Autodesk Inventor part; units mm, degrees
ref_plane "YZ Plane" through (0, 0, 0) normal (1, 0, 0) x (0, 1, 0)
ref_plane "XZ Plane" through (0, 0, 0) normal (0, 1, 0) x (-1, 0, 0)
ref_plane "XY Plane" through (0, 0, 0) normal (0, 0, 1) x (1, 0, 0)
sketch "Sketch1" plane through (0, 0, 0) normal (0, 1, 0) x (-1, 0, 0)
  line L0 (10.07, 20.05) -> (-10.07, 20.05)
  line L1 (-10.07, 20.05) -> (-10.07, -20.05)
  line L2 (-10.07, -20.05) -> (10.07, -20.05)
  line L3 (10.07, -20.05) -> (10.07, 20.05)
  point P0 (0, 0)
  dimension "d0" = 40.1
  dimension "d1" = 20.14
  dimension "d2" = 10.07
  dimension "d3" = 20.05
extrude "Plate1" add sketch "Sketch1" along normal blind 1.5
sketch "Sketch2" plane through (10.07, 0, 21.55) normal (0, 0, -1) x (-1, 0, 0)
  line L0 (20.14, 0) -> (0, 0)
  line L1 (0, 0) -> (0, 60)
  line L2 (0, 60) -> (20.14, 60)
  line L3 (20.14, 60) -> (20.14, 0)
edge flange "Flange1" height 60 angle 90 thickness 1.5 bend radius 0.31 thickness toward (0, 0, -1) relief tear relief width 1.5 relief depth 0.75 corner gap 0.31 corner form 0 edges at (0, 1.5, 20.05) (0, 1.5, -20.05) wall of the first edge with corners at (-10.07, 0, 21.55) (10.07, 0, 21.55) (10.07, 60, 21.55) (-10.07, 60, 21.55)
bend "Bend1"
corner "Corner1"
sketch "Sketch15" plane through (10.07, 60, -21.55) normal (0, 0, -1) x (-1, 0, 0)
  circle A0 centre (2.545, -12.76) radius 0.7835
  circle A1 centre (17.595, -12.76) radius 0.7835
  circle A2 centre (2.545, -27.86) radius 0.7835
  circle A3 centre (17.595, -27.86) radius 0.7835
  point P0 (10.07, -60)
hole "Hole9" at (7.525, 47.24, -21.55) at (-7.525, 47.24, -21.55) at (7.525, 32.14, -21.55) at (-7.525, 32.14, -21.55) direction (0, 0, 1) diameter 2.1 depth 1.5
sketch "Sketch16" plane through (-10.07, 60, 21.55) normal (0, 0, 1) x (1, 0, 0)
  circle A0 centre (18.07, -7.16) radius 0.7835
  circle A1 centre (2.07, -7.16) radius 0.7835
  circle A2 centre (3.07, -20.38) radius 0.7835
  circle A3 centre (17.07, -20.38) radius 0.7835
  circle A4 centre (10.07, -27.68) radius 0.7835
  point P0 (10.07, -60)
hole "Hole10" at (-8, 52.84, 21.55) at (8, 52.84, 21.55) at (-7, 39.62, 21.55) at (7, 39.62, 21.55) at (0, 32.32, 21.55) direction (0, 0, -1) diameter 2.1 depth 1.5
sketch "Sketch17" plane through (-10.07, 60, 21.55) normal (0, 0, 1) x (1, 0, 0)
  point P0 (10.07, -60)
sketch "Sketch18" plane through (-10.07, 60, 21.55) normal (0, 0, 1) x (1, 0, 0)
  point P0 (10.07, -60)
sketch "Sketch19" plane through (-10.07, 60, 21.55) normal (0, 0, 1) x (1, 0, 0)
  circle A0 centre (10.07, -0.26) radius 6
  point P0 (10.07, -60)
sketch "Sketch20" plane through (10.07, 60, -21.55) normal (0, 0, -1) x (-1, 0, 0)
  circle A0 centre (10.07, -0.26) radius 6
  point P0 (10.07, -60)
sketch "Sketch21" plane through (0, 0, 0) normal (0, -1, 0) x (1, 0, 0)
  circle A0 centre (4.76, 2.25) radius 1.5
  circle A1 centre (4.76, -13.05) radius 1.5
  circle A2 centre (-5.38, -13.05) radius 1.5
  circle A3 centre (-5.38, 2.25) radius 1.5
  point P0 (0, 0)
fillet "Corner Round1" radius 1 4 edges at (-10.07, 60, 20.8) (-10.07, 60, -20.8) (10.07, 60, -20.8) (10.07, 60, 20.8)
hole "Hole11" at (-5.38, 0, -13.05) at (4.76, 0, -13.05) at (-5.38, 0, 2.25) at (4.76, 0, 2.25) direction (0, 1, 0) diameter 3.1 depth 1.5
hole "Hole12" at (0, 59.74, 21.55) direction (0, 0, -1) diameter 13.5 depth 1.5
hole "Hole13" at (0, 59.74, -21.55) direction (0, 0, 1) diameter 13.5 depth 1.5
equation "\"d96\" = Thickness"
equation "\"d103\" = Thickness"
equation "\"d117\" = Thickness"
equation "\"d124\" = Thickness"
equation "\"d131\" = Thickness"
equation "\"d4\" = Thickness"
equation "\"d5\" = BendReliefWidth"
equation "\"d6\" = BendReliefDepth"
equation "\"d7\" = MinimumRemnant"
equation "\"d8\" = TransitionRadius"
equation "\"d11\" = BendRadius"
equation "\"d12\" = CornerReliefSize"
equation "\"d13\" = GapSize"
equation "\"d14\" = JacobiRadiusSize"
equation "\"BendReliefWidth\" = Thickness"
equation "\"BendReliefDepth\" = 0.5 * Thickness"
equation "\"CornerReliefSize\" = 4 * Thickness"
equation "\"MinimumRemnant\" = 2 * Thickness"
equation "\"TransitionRadius\" = BendRadius"
equation "\"JacobiRadiusSize\" = BendRadius"
equation "\"GapSize\" = Thickness"
properties part number "axis_25_top_frame" material "Aluminum 6061-AHC"
Here's how the part is built. I have some questions about the finished solid (model axes, mm). A direction names the side the tool comes from. Give positions to 0.01 mm unless a question says otherwise; leave off trailing zeros. Write each loop counter-clockwise with the first axis right and the second up, starting at its lowest first coordinate (ties: lowest second). Pieces come first, ordered by that corner, then holes. Notation, with made-up numbers: M 47,81 L 62,81 A11 ccw 62,100 Z; hole C 86.25,48 d4. An arc over 180 degrees is marked long. Put each result on its own line as item: value. Start each with the question number.
Item 1: Thinking about a two-plate mould opening in Y: for faces 1 (the cylindrical face through (4.294, 0.76, -14.528)), 2 (the flat face through (-8, 60, 21)), 3 (the cylindrical face through (7.48, 31.09, -20.79)), 4 (the cylindrical face through (-0.05, 33.37, 20.79)), which applies, +Y half, -Y half, draft (parallel to the pull), parting line (faces both ways), or undercut?
Item 2: If we section it at B-B, the plane x = 0: Write out the boundary of the cut face in (y, z).
Item 3: Will these pins go through, and if not, where does the flat tip stop? pin 1 (5 mm diameter, centred on x = -5.38, z = 2.25, fed in from -Y); pin 2 (1.9 mm diameter, centred on x = 8, y = 52.84, fed in from +Z); pin 3 (4 mm diameter, centred on x = 3.5, z = -16.5, fed in from +Y).
Item 4: If we section it at A-A, the plane y = 14: Write out the boundary of the cut face in (x, z).
Item 5: If we section it at C-C, the plane y = 47.24: Write out the boundary of the cut face in (x, z) (3 decimals), then the cut area to 3 significant figures.
Item 6: If we section it at D-D, the plane z = 2.5: Write out the boundary of the cut face in (x, y), then the cut area to 3 significant figures.
Item 7: I need wall thicknesses on L1, parallel to X at y = 0.4, z = -13.05; L2, parallel to Z at x = -2.25, y = 42; L3, parallel to X at y = 47.24, z = -20.8 (3 decimals). Which ranges of each line are inside material? Lowest first, please. Write a range as from..to.
Item 8: On a 3-axis mill with a long thin cutter (end or side, diameter ignored), from which of +Z, -Z, +X, -X, +Y, -Y can I reach the whole of each face in a straight line? I mean faces 5 (the cylindrical face through (-8.9, 52.3, 20.8)), 6 (the flat face through (0, 1.5, 0)), 7 (the cylindrical face through (0.14, 0.54, 21.03)), 8 (the cylindrical face through (-7.57, 31.09, -20.79)), 9 (the flat face through (8, 60, -21)). Say none if no direction works.
Values:
1. face 1: draft
1. face 2: +Y half
1. face 3: undercut
1. face 4: undercut
2. outline: M 0,-19.74 A1.81 ccw 1.81,-21.55 L 52.99,-21.55 L 52.99,-20.05 L 1.81,-20.05 A0.31 cw 1.5,-19.74 L 1.5,19.74 A0.31 cw 1.81,20.05 L 31.27,20.05 L 31.27,21.55 L 1.81,21.55 A1.81 ccw 0,19.74 Z; M 33.37,20.05 L 52.99,20.05 L 52.99,21.55 L 33.37,21.55 Z
3. pin 1: y = 0
3. pin 2: z = -20.05
3. pin 3: y = 1.5
4. outline: M -10.07,-21.55 L 10.07,-21.55 L 10.07,-20.05 L -10.07,-20.05 Z; M -10.07,20.05 L 10.07,20.05 L 10.07,21.55 L -10.07,21.55 Z
5. outline: M -10.07,-21.55 L -8.575,-21.55 L -8.575,-20.05 L -10.07,-20.05 Z; M -10.07,20.05 L 10.07,20.05 L 10.07,21.55 L -10.07,21.55 Z; M -6.475,-21.55 L 6.475,-21.55 L 6.475,-20.05 L -6.475,-20.05 Z; M 8.575,-21.55 L 10.07,-21.55 L 10.07,-20.05 L 8.575,-20.05 Z
5. area: 54.1 mm²
6. outline: M -10.07,0 L -6.91,0 L -6.91,1.5 L -10.07,1.5 Z; M -3.85,0 L 3.23,0 L 3.23,1.5 L -3.85,1.5 Z; M 6.29,0 L 10.07,0 L 10.07,1.5 L 6.29,1.5 Z
6. area: 21.0 mm²
7. L1: -10.07..-6.93, -3.83..3.21, 6.31..10.07
7. L2: -21.55..-20.05, 20.05..21.55
7. L3: -10.07..-8.575, -6.475..6.475, 8.575..10.07
8. face 5: +Z
8. face 6: +X, -X, +Y
8. face 7: +Z, +X, -X, -Y
8. face 8: -Z
8. face 9: +Z, -Z, +X, -X, +Y
